from build123d import *

# Parameters (mm, degrees)
SKETCH1_R           = 3
BOSS_EXTRUDE1_DEPTH = 6
SCALE1_SCALE        = 0.5


with BuildPart() as part:
    # Sketch1 → Boss-Extrude1 (new body)
    with BuildSketch(Plane.XY):
        with BuildLine():
            Line((6, 17.5), (6, -17.5))
            ThreePointArc((6, -17.5), (0, -23.5), (-6, -17.5))
            Line((-6, -17.5), (-6, 17.5))
            ThreePointArc((-6, 17.5), (0, 23.5), (6, 17.5))
        make_face()
        with Locations((0, 17.5)):
            Circle(SKETCH1_R, mode=Mode.SUBTRACT)
        with Locations((0, -17.5)):
            Circle(SKETCH1_R, mode=Mode.SUBTRACT)
    extrude(amount=-BOSS_EXTRUDE1_DEPTH)


with BuildPart() as part_1:
    # Scale1: scaled about (0, 0, -3)
    add(part.part.scale(SCALE1_SCALE).moved(Location((0, 0, -1.5))))


solid = part_1.part
Can you work these out from the model? Positions are in its coordinate system, mm. Coordinates: 2 decimals unless noted, no trailing zeros. Loops run counter-clockwise (first coordinate to the right, second up) from the corner with the lowest first, then second, coordinate; pieces in that order, holes last. Notation, with made-up numbers: (14, 81) - (64, 81) arc R19 ccw to (64, 102) - close; hole circle Ø8 at (-13, 89). An arc over 180 degrees is marked (long way). Answer as a JSON object with one key per item and string values. Group by question number.
Item 1: If we section it at D-D (x = -2.55): List the corners of the cut face in (y, z) for me, plus the area to 3 significant figures.
Item 2: If I drill on L1, parallel to Y at x = 0, z = -3.55; L2, parallel to Y at x = -0.6, z = -2.9; L3, parallel to X at y = 8.5, z = -2.45, over which ranges is the centre line in solid material (lowest first)? Write a range as from..to.
Item 3: If we mould it in two halves opening along X, with no side actions, what happens to faces 1 (the face through (-3, 0, -3)), 2 (the face through (0.07, -11.75, -2.98)), 3 (the face through (-0.325, -10.214, -2.979))? For each: released by +X, released by -X, zero draft, split by the parting line, or undercut.
Item 4: For pin 1 (2.5 mm diameter, centred on x = 0, y = 8.75, fed in from +Z), with a flat end and sliding along its axis, tell me the tip position at first contact or that it passes through.
Item 5: If we section it at C-C (x = 1.25): List the corners of the cut face in (y, z) for me, plus the area to 3 significant figures.
Item 6: If we section it at A-A (x = 0): List the corners of the cut face in (y, z) for me.
Item 7: If we section it at B-B (z = -3.45): List the corners of the cut face in (x, y) for me.
Returned:
{
 "1": {"outline": "(-10.33, -4.5) - (10.33, -4.5) - (10.33, -1.5) - (-10.33, -1.5) - close", "area": "62.0 mm²"},
 "2": {"L1": "y = -11.75..-10.25, -7.25..7.25, 10.25..11.75", "L2": "y = -11.69..-10.12, -7.38..7.38, 10.12..11.69", "L3": "x = -3..-1.48, 1.48..3"},
 "3": {"face 1": "released by -X", "face 2": "split by the parting line", "face 3": "undercut"},
 "4": {"pin 1": "passes through"},
 "5": {"outline": "(-11.48, -4.5) - (-9.58, -4.5) - (-9.58, -1.5) - (-11.48, -1.5) - close; (-7.92, -4.5) - (7.92, -4.5) - (7.92, -1.5) - (-7.92, -1.5) - close; (9.58, -4.5) - (11.48, -4.5) - (11.48, -1.5) - (9.58, -1.5) - close", "area": "58.9 mm²"},
 "6": {"outline": "(-11.75, -4.5) - (-10.25, -4.5) - (-10.25, -1.5) - (-11.75, -1.5) - close; (-7.25, -4.5) - (7.25, -4.5) - (7.25, -1.5) - (-7.25, -1.5) - close; (10.25, -4.5) - (11.75, -4.5) - (11.75, -1.5) - (10.25, -1.5) - close"},
 "7": {"outline": "(-3, -8.75) arc R3 ccw to (3, -8.75) - (3, 8.75) arc R3 ccw to (-3, 8.75) - close; hole circle Ø3 at (0, -8.75); hole circle Ø3 at (0, 8.75)"}
}
